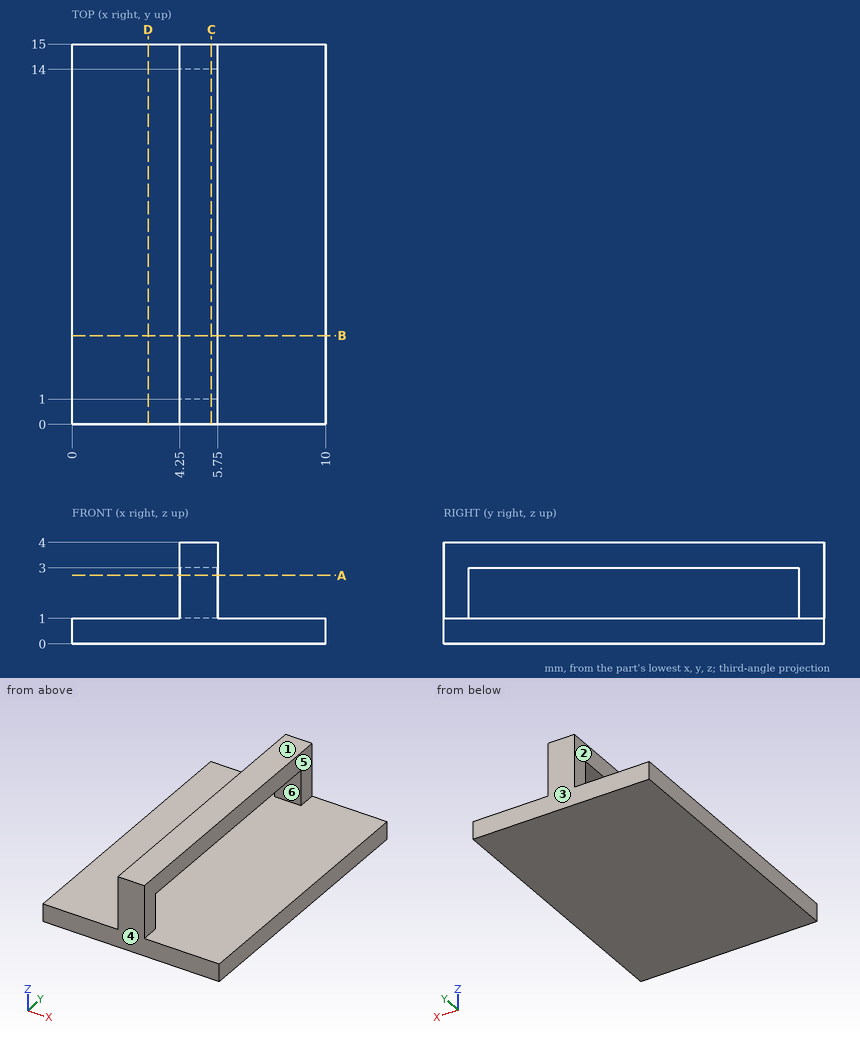
Study the drawing (mm; zero at the part's minimum x, y, z) and answer. A direction names the side the tool comes from. Round coordinates to 2 decimals unless told otherwise and drop trailing zeros. Write each loop counter-clockwise with the first axis right and the second up, starting at its lowest first coordinate (ties: lowest second). Pieces come first, ordered by that corner, then holes. Notation, with made-up numbers: (16, 18) - (33, 18) arc R17 cw to (33, 38) - close; hole circle Ø4 at (-28.5, 81.5). An arc over 180 degrees is marked (long way). Use a Markdown table: item, result. Add a question column.
1. Flat-ended cylindrical pins translate along their axes: P1, Ø3, axis at x = 1.5, y = 8, coming from the +Z side; P2, Ø0.9, axis at y = 7.5, z = 2.5, coming from the -X side. Find the tip coordinate at first contact, or state that the pin passes through.
2. Consider line 1 (Z direction, x = 1.75, y = 12.5); line 2 (X direction, y = 4.25, z = 3.1). Determine where each line is inside the solid, lowest interval first.
3. For a pull along Y with two mould halves and no side action, classify the marked faces 3, 4, 5 and 6 as +Y half, -Y half, draft (parallel to the pull), parting line (faces both ways), or undercut.
4. The part is cut by section D-D (x = 3). Write down the section's boundary in (y, z).
5. A tool of negligible diameter and unlimited length cuts with its end or side. For the marked faces 1 and 2, from which of +Z, -Z, +X, -X, +Y, -Y can it reach the whole face along a straight path? Write none if from no direction.
6. The part is cut by section B-B (y = 3.5). Write down the section's boundary in (x, z), and give its area (3 significant figures).
7. The part is cut by section C-C (x = 5.5). Write down the section's boundary in (y, z).
8. The part is cut by section A-A (z = 2.7). Write down the section's boundary in (x, y).
Reported:
| question | item | result |
|---|---|---|
| 1 | P1 | z = 1 |
| 1 | P2 | through |
| 2 | line 1 | 0 to 1 |
| 2 | line 2 | 4.25 to 5.75 |
| 3 | face 3 | +Y half |
| 3 | face 4 | -Y half |
| 3 | face 5 | draft |
| 3 | face 6 | undercut |
| 4 | outline | (0, 0) - (15, 0) - (15, 1) - (0, 1) - close |
| 5 | face 1 | +Z, +X, -X, +Y, -Y |
| 5 | face 2 | +Z, -X, +Y, -Y |
| 6 | outline | (0, 0) - (10, 0) - (10, 1) - (0, 1) - close; (4.25, 3) - (5.75, 3) - (5.75, 4) - (4.25, 4) - close |
| 6 | area | 11.5 mm^2 |
| 7 | outline | (0, 0) - (15, 0) - (15, 4) - (0, 4) - close; hole (1, 1) - (14, 1) - (14, 3) - (1, 3) - close |
| 8 | outline | (4.25, 0) - (5.75, 0) - (5.75, 1) - (4.25, 1) - close; (4.25, 14) - (5.75, 14) - (5.75, 15) - (4.25, 15) - close |
